The listing builds one solid part. Answer for the finished solid, in the listing's coordinates (mm). A direction names the side the tool comes from. Round coordinates to 2 decimals unless told otherwise and drop trailing zeros. Write each loop counter-clockwise with the first axis right and the second up, starting at its lowest first coordinate (ties: lowest second). Pieces come first, ordered by that corner, then holes.
(1) A cutting plane is placed at A-A, the plane y = 14.5. Give the vertices of the cut face in (x, z).
(2) For faces 5 (the face through (159, 0, 9)), 6 (the face through (2, 3.81, 9)), 7 (the face through (163, 3.81, 9)), determine the directions among +Z, -Z, +X, -X, +Y, -Y from which every point of the face is accessible in a straight line to the end or side of a thin tool.
(3) Find the intervals of material crossed by probe 1 along X at (y, z) = (3, 1.5); probe 2 along X at (y, z) = (19.5, 1.75); probe 3 along Y at (x, z) = (57.5, 13.75), in increasing order.
(4) Each of these flat-tipped pins is pushed along its axis until it touches: pin 1 Ø5 at (x, z) = (128, 6.5) entering from +Y; pin 2 Ø1.9 at (x, z) = (2, 13.5) entering from +Y; pin 3 Ø1.5 at (x, z) = (105.5, 3.5) entering from -Y. Where does it stop, or does it pass through?
(5) A cutting plane is placed at D-D, the plane x = 53.5. Give the vertices of the cut face in (y, z).
(6) The mould has two halves that part along X. Classify faces 1 (the face through (127.352, 33.252, 9.392)), 2 (the face through (12.7, 2, 9)), 3 (the face through (152.4, 2, 9)), 4 (the face through (6, 0, 9)): +X half, -X half, draft (parallel to the pull), parting line (faces both ways), or undercut.
(7) A cutting plane is placed at C-C, the plane y = 25. Give the vertices of the cut face in (x, z), and give its area (3 significant figures).
(8) A cutting plane is placed at B-B, the plane z = 5.5. Give the vertices of the cut face in (x, y), and give its area (3 significant figures).
from build123d import *

# Parameters (mm, degrees)
BOSS_EXTRUDE1_DEPTH = 19.05


with BuildPart() as part:
    # Sketch1 → Boss-Extrude1 (new body)
    with BuildSketch(Plane.XY):
        with BuildLine():
            Line((0, 0), (12.7, 0))
            Line((12.7, 0), (12.7, 3.81))
            Line((12.7, 3.81), (10.16, 3.81))
            ThreePointArc((10.16, 3.81), (42.442039197, 29.215695028), (82.55, 38.1))
            ThreePointArc((82.55, 38.1), (122.657960803, 29.215695028), (154.94, 3.81))
            Line((154.94, 3.81), (152.4, 3.81))
            Line((152.4, 3.81), (152.4, 0))
            Line((152.4, 0), (165.1, 0))
            Line((165.1, 0), (165.1, 3.81))
            Line((165.1, 3.81), (161.29, 3.81))
            ThreePointArc((161.29, 3.81), (126.781281636, 33.54873317), (82.55, 44.45))
            ThreePointArc((82.55, 44.45), (38.318718364, 33.54873317), (3.81, 3.81))
            Line((3.81, 3.81), (0, 3.81))
            Line((0, 3.81), (0, 0))
        make_face()
    extrude(amount=BOSS_EXTRUDE1_DEPTH)


solid = part.part
Solutions:
1. outline: (12.74, 0) - (20.31, 0) - (20.31, 19.05) - (12.74, 19.05) - close; (144.79, 0) - (152.36, 0) - (152.36, 19.05) - (144.79, 19.05) - close
2. face 5: +Z, -Z, +X, -X, -Y
2. face 6: +Z, -Z, -X, +Y
2. face 7: +Z, -Z, +X, +Y
3. probe 1: x = 0 to 12.7, 152.4 to 165.1
3. probe 2: x = 17.93 to 26.39, 138.71 to 147.17
3. probe 3: y = 34.8 to 41.01
4. pin 1: stops at y = 34.2
4. pin 2: stops at y = 3.81
4. pin 3: stops at y = 35.16
5. outline: (33.61, 0) - (39.83, 0) - (39.83, 19.05) - (33.61, 19.05) - close
6. face 1: +X half
6. face 2: undercut
6. face 3: undercut
6. face 4: draft
7. outline: (24.65, 0) - (34.55, 0) - (34.55, 19.05) - (24.65, 19.05) - close; (130.55, 0) - (140.45, 0) - (140.45, 19.05) - (130.55, 19.05) - close
7. area: 377 mm2
8. outline: (0, 0) - (12.7, 0) - (12.7, 3.81) - (10.16, 3.81) arc R92.31 cw to (82.55, 38.1) arc R92.31 cw to (154.94, 3.81) - (152.4, 3.81) - (152.4, 0) - (165.1, 0) - (165.1, 3.81) - (161.29, 3.81) arc R97.9 ccw to (82.55, 44.45) arc R97.9 ccw to (3.81, 3.81) - (0, 3.81) - close
8. area: 1,090 mm2
